Verification items for the finished model (mm, model axes). Face numbers are marked on the shaded views. A direction names the side the tool comes from. Round coordinates to 2 decimals unless told otherwise and drop trailing zeros. Loops run counter-clockwise (first coordinate to the right, second up) from the corner with the lowest first, then second, coordinate; pieces in that order, holes last. Notation, with made-up numbers: (44, 16.5) -> (80, 16.5) arc R16 cw to (80, 44.5) -> close; hole circle Ø9 at (34, 81). An arc over 180 degrees is marked (long way). Write item = value, one per line. Start each with the question number.
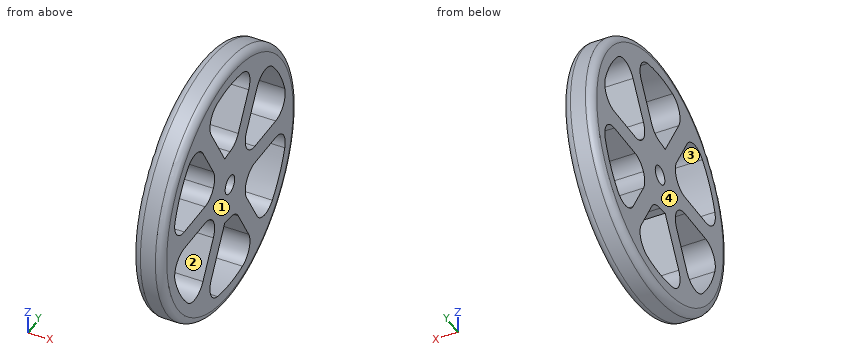
Autodesk Inventor part; units mm, degrees
ref_plane "YZ Plane" through (0, 0, 0) normal (1, 0, 0) x (0, 1, 0)
ref_plane "XZ Plane" through (0, 0, 0) normal (0, 1, 0) x (-1, 0, 0)
ref_plane "XY Plane" through (0, 0, 0) normal (0, 0, 1) x (1, 0, 0)
sketch "Esboço1" plane through (0, 0, 0) normal (1, 0, 0) x (0, 1, 0)
  circle A0 centre (0, 0) radius 35
  circle A1 centre (0, 0) radius 2.5
  line L0 (9.6825, 2.5) -> (29.8957, 2.5)
  line L1 (29.8957, -2.5) -> (9.6825, -2.5)
  line L2 (17.1129, 24.6404) -> (7.0063, 7.1353)
  line L3 (2.6762, 9.6353) -> (12.7828, 27.1404)
  line L4 (-12.7828, 27.1404) -> (-2.6762, 9.6353)
  line L5 (-7.0063, 7.1353) -> (-17.1129, 24.6404)
  line L6 (-29.8957, 2.5) -> (-9.6825, 2.5)
  line L7 (-9.6825, -2.5) -> (-29.8957, -2.5)
  line L8 (-17.1129, -24.6404) -> (-7.0063, -7.1353)
  line L9 (-2.6762, -9.6353) -> (-12.7828, -27.1404)
  line L10 (12.7828, -27.1404) -> (2.6762, -9.6353)
  line L11 (7.0063, -7.1353) -> (17.1129, -24.6404)
  arc A2 (29.8957, 2.5) -> (17.1129, 24.6404) centre (0, 0) ccw
  arc A3 (12.7828, 27.1404) -> (-12.7828, 27.1404) centre (0, 0) ccw
  arc A4 (-17.1129, 24.6404) -> (-29.8957, 2.5) centre (0, 0) ccw
  arc A5 (-29.8957, -2.5) -> (-17.1129, -24.6404) centre (0, 0) ccw
  arc A6 (-12.7828, -27.1404) -> (12.7828, -27.1404) centre (0, 0) ccw
  arc A7 (17.1129, -24.6404) -> (29.8957, -2.5) centre (0, 0) ccw
  arc A8 (-2.6762, -9.6353) -> (2.6762, -9.6353) centre (0, 0) ccw
  arc A9 (2.6762, 9.6353) -> (-2.6762, 9.6353) centre (0, 0) ccw
  arc A10 (7.0063, -7.1353) -> (9.6825, -2.5) centre (0, 0) ccw
  arc A11 (9.6825, 2.5) -> (7.0063, 7.1353) centre (0, 0) ccw
  arc A12 (-7.0063, 7.1353) -> (-9.6825, 2.5) centre (0, 0) ccw
  arc A13 (-9.6825, -2.5) -> (-7.0063, -7.1353) centre (0, 0) ccw
  dimension "d0" = 70
  dimension "d3" = 5
  dimension "d4" = 5
  dimension "d5" = 2.5
  dimension "d8" = 360
  dimension "d10" = 30
  dimension "d11" = 10
extrude "Extrusão1" add sketch "Esboço1" along normal mid plane 8
fillet "Arredondamento1" radius 2 2 edges at (-4, -35, 0) (4, -35, 0)
fillet "Arredondamento2" radius 5 44 edges at (2, 12.7828, -27.1404) (-2, 12.7828, -27.1404) (2, 17.1129, -24.6404) (-2, 17.1129, -24.6404) (2, 29.8957, 2.5) (-2, 29.8957, 2.5) (2, 29.8957, -2.5) (-2, 29.8957, -2.5) (2, 2.6762, -9.6353) (-2, 2.6762, -9.6353) (2, 7.0063, -7.1353) (-2, 7.0063, -7.1353) (2, 9.6825, -2.5) (-2, 9.6825, -2.5) (2, 9.6825, 2.5) (-2, 9.6825, 2.5) (2, 7.0063, 7.1353) (-2, 7.0063, 7.1353) (2, 17.1129, 24.6404) (-2, 17.1129, 24.6404) (2, 12.7828, 27.1404) (-2, 12.7828, 27.1404) (2, -7.0063, 7.1353) (-2, -7.0063, 7.1353) (2, -9.6825, 2.5) (-2, -9.6825, 2.5) (2, 2.6762, 9.6353) (-2, 2.6762, 9.6353) (2, -7.0063, -7.1353) (-2, -7.0063, -7.1353) (2, -9.6825, -2.5) (-2, -9.6825, -2.5) (2, -12.7828, 27.1404) (-2, -12.7828, 27.1404) (2, -17.1129, 24.6404) (-2, -17.1129, 24.6404) (2, -29.8957, -2.5) (-2, -29.8957, -2.5) (2, -29.8957, 2.5) (-2, -29.8957, 2.5) (2, -12.7828, -27.1404) (-2, -12.7828, -27.1404) (2, -17.1129, -24.6404) (-2, -17.1129, -24.6404)
properties part number "Wheel"
(1) Section check A-A on z = 0. Enter the section's corners in (x, y), then the cut area to 3 significant figures.
(2) Draft check along Z on the marked faces 1 and 2. Enter one of: +Z half, -Z half, draft (parallel to the pull), parting line (faces both ways), or undercut.
(3) Access from +Z, -Z, +X, -X, +Y, -Y to the whole of each face (thin tool, end or side, straight path). Record for the marked faces 3 and 4.
(4) Scan lines: line 1 (Z direction, x = 0.5, y = 0); line 2 (Z direction, x = -0.25, y = -26); line 3 (Y direction, x = 0, z = 10.5). Record each from-to range of solid material in increasing order. Write a range as [from, to].
(5) Section check B-B on x = 0. Give the number of separate pieces and of enclosed holes in the cut face, then the cut area to 3 significant figures.
(6) Depth check by flat-ended pin: pin 1 Ø1 at (x, z) = (0.5, -19.5) entering from -Y; pin 2 Ø4 at (x, y) = (2, 17) entering from -Z; pin 3 Ø1.5 at (y, z) = (-0.5, -11.5) entering from -X; pin 4 Ø1.5 at (x, z) = (-3, 23.5) entering from +Y. Enter the tip coordinate at first touch or a pass-through.
Computed values:
q1.outline = (-4, -33) arc R2 ccw to (-2, -35) -> (2, -35) arc R2 ccw to (4, -33) -> (4, -2.5) -> (-4, -2.5) -> close; (-4, 2.5) -> (4, 2.5) -> (4, 33) arc R2 ccw to (2, 35) -> (-2, 35) arc R2 ccw to (-4, 33) -> close
q1.area = 517 mm²
q2.face_1 = draft
q2.face_2 = undercut
q3.face_3 = +X, -X
q3.face_4 = +Z, -Z, -X, +Y, -Y
q4.line_1 = [-35, -30], [-10, -2.5], [2.5, 10], [30, 35]
q4.line_2 = [-23.43, -14.97], [-2.99, 2.99], [14.97, 23.43]
q4.line_3 = [-33.39, -28.1], [-8.95, -3.18], [2.18, 8.95], [28.1, 33.39]
q5.separate_pieces = 1
q5.enclosed_holes = 7
q5.area = 2,040 mm²
q6.pin_1 = -29.39
q6.pin_2 = -31.62
q6.pin_3 = through
q6.pin_4 = 26.38
